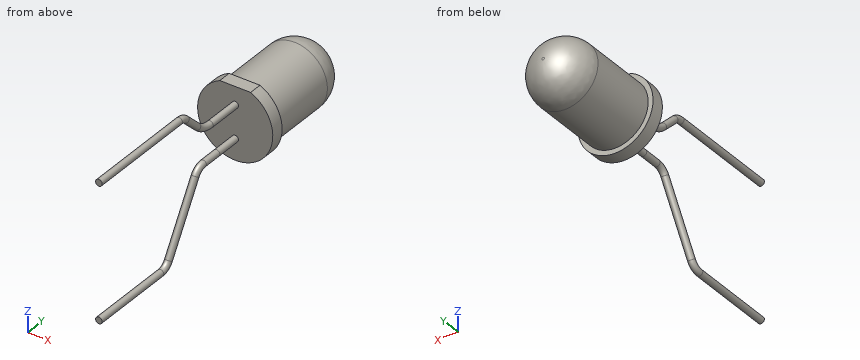
from build123d import *

# Parameters (mm, degrees)
CUT_EXTRUDE1_DEPTH  = 1
SKETCH3_R           = 0.25
BOSS_EXTRUDE1_DEPTH = 2
SKETCH5_R           = 0.25
SKETCH7_R           = 0.25


with BuildPart() as part:
    # Sketch1 → Revolve1 (revolve)
    with BuildSketch(Plane.XY, mode=Mode.PRIVATE) as revolve1_sk:
        with BuildLine():
            Line((0, 0), (0, 8.75))
            Line((0, 8.75), (0.1, 8.75))
            ThreePointArc((0.1, 8.75), (1.782914139, 8.052914139), (2.48, 6.37))
            Line((2.48, 6.37), (2.48, 1))
            Line((2.48, 1), (2.85, 1))
            Line((2.85, 1), (2.85, 0))
            Line((2.85, 0), (0, 0))
        make_face()
    revolve(revolve1_sk.sketch.rotate(Axis((0, 0, 0), (0, 1, 0)), 90), axis=Axis((0, 0, 0), (0, 1, 0)))

    # Sketch2 → Cut-Extrude1 (cut)
    with BuildSketch(Plane.XZ):
        with BuildLine():
            Line((-1.167261753, 2.6), (1.167261753, 2.6))
            ThreePointArc((1.167261753, 2.6), (0, 2.85), (-1.167261753, 2.6))
        make_face()
    extrude(amount=-CUT_EXTRUDE1_DEPTH, mode=Mode.SUBTRACT)

    # Sketch3 → Boss-Extrude1 (add)
    with BuildSketch(Plane.XZ):
        with Locations(Location((0, -1.25, 0), (0, 0, 270))):
            Circle(SKETCH3_R)
        with Locations(Location((0, 1.25, 0), (0, 0, 270))):
            Circle(SKETCH3_R)
    extrude(amount=BOSS_EXTRUDE1_DEPTH)

    # Sweep1: sweep along a path in Sketch4
    with BuildLine(Plane(origin=(0, 0, 0), x_dir=(0, 0, -1), z_dir=(1, 0, 0))) as sweep1_path:
        Line((-1.25, -2), (-1.25, -2.7))
        ThreePointArc((-1.25, -2.7), (-1.393046618, -3.442781353), (-1.801724138, -4.079310345))
        Line((-1.801724138, -4.079310345), (-2.974137931, -5.310344828))
        ThreePointArc((-2.974137931, -5.310344828), (-3.178476691, -5.628609324), (-3.25, -6))
        Line((-3.25, -6), (-3.25, -14.6))
    # Sketch5 → Sweep1 (sweep)
    with BuildSketch(Plane(origin=(0, -14.6, 3.25), x_dir=(-1, 0, 0), z_dir=(0, -1, 0))):
        Circle(SKETCH5_R)
    sweep(path=sweep1_path.line)

    # Sweep2: sweep along a path in Sketch6
    with BuildLine(Plane(origin=(0, 0, 0), x_dir=(0, 0, -1), z_dir=(1, 0, 0))) as sweep2_path:
        Line((6.91, -14.6), (6.91, -8))
        ThreePointArc((6.91, -8), (6.78151551, -7.50963206), (6.429078567, -7.14527347))
        Line((6.429078567, -7.14527347), (1.730921433, -4.292065356))
        ThreePointArc((1.730921433, -4.292065356), (1.37848449, -3.927706766), (1.25, -3.437338826))
        Line((1.25, -3.437338826), (1.25, -2))
    # Sketch7 → Sweep2 (sweep)
    with BuildSketch(Plane(origin=(0, -14.6, -6.91), x_dir=(-1, 0, 0), z_dir=(0, -1, 0))):
        Circle(SKETCH7_R)
    sweep(path=sweep2_path.line)


solid = part.part
Can you work these out from the model? Positions are in its coordinate system, mm. Coordinates: 2 decimals unless noted, no trailing zeros. Loops run counter-clockwise (first coordinate to the right, second up) from the corner with the lowest first, then second, coordinate; pieces in that order, holes last. Notation, with made-up numbers: (84.5, 18.25) - (118.5, 18.25) arc R17 cw to (118.5, 43.25) - close; hole circle Ø1 at (25, 19.5). An arc over 180 degrees is marked (long way). Answer as a JSON object with one key per item and string values. Group by question number.
Item 1: If I drill on L1, parallel to Y at x = 1.7, z = 2; L2, parallel to Z at x = 0.2, y = -2.25; L3, parallel to Y at x = -1.3, z = 0.75, over which ranges is the centre line in solid material (lowest first)? Write a range as from..to.
Item 2: For pin 1 (1 mm diameter, centred on x = 1.5, y = 3, fed in from -Z); pin 2 (4 mm diameter, centred on y = 2, z = -3, fed in from +X), each with a flat end and sliding along its axis, tell me the tip position at first contact or that it passes through.
Item 3: If we section it at A-A (y = -9): List the corners of the cut face in (x, z) for me.
Returned:
{
 "1": {"L1": "y = 0..1", "L2": "z = -1.4..-1.1, 1.1..1.4", "L3": "y = 0..8.29"},
 "2": {"pin 1": "stops at z = -2.27", "pin 2": "stops at x = 2.55"},
 "3": {"outline": "circle Ø0.5 at (0, -6.91); circle Ø0.5 at (0, 3.25)"}
}
